Geometry check sheet. Reference: the model listing, model coordinates, mm. A direction names the side the tool comes from. Coordinates: 2 decimals unless noted, no trailing zeros. Write each loop counter-clockwise with the first axis right and the second up, starting at its lowest first coordinate (ties: lowest second). Pieces come first, ordered by that corner, then holes. Notation, with made-up numbers: (-12, 49.5) -> (47, 49.5) arc R12 cw to (47, 68.5) -> close; hole circle Ø10 at (44, 38.5). An arc over 180 degrees is marked (long way). Answer in a Markdown table with one row per item. Add a question column.
Q1. Section check B-B, the plane y = 15. Record the boundary of the cut face in (x, z), and give its area (3 significant figures).
Q2. Section check A-A, the plane z = -6.25. Record the boundary of the cut face in (x, y), and give its area (3 significant figures).
Q3. Tool access check on faces 1 (the face through (-27.488, -47.465, 0.246)), 2 (the face through (-21.883, 55.465, -9.616)), 3 (the face through (-29, 58, -8)), 4 (the face through (-25, 54, -21)), 5 (the face through (-24, -45, 0)). Record the directions out of +Z, -Z, +X, -X, +Y, -Y that give a thin tool (end or side, any length) a straight path to the whole face; none if there is none.
Q4. Thickness scan on line 1 (X direction, y = 54.45, z = 0); line 2 (Y direction, x = -26.5, z = -14); line 3 (Y direction, x = -21, z = -3.5). Record the ranges inside material, lowest first.
Q5. Release check for a two-part mould opening along Z. For faces 6 (the face through (-25, -50, 0)), 7 (the face through (-28.905, 3.165, 0.867)), 8 (the face through (-25, 55, -19)) record: pulls with the +Z half, pulls with the -Z half, needs draft (parallel to the pull), parting line crosses it, or undercut.
Q6. Gauge pin test, flat ends, axial feed: P1, Ø1.5, axis at y = -16.5, z = 0.5, coming from the +X side; P2, Ø12, axis at y = 7.5, z = -7, coming from the -X side; P3, Ø1.1, axis at x = -22, y = 6, coming from the -Z side; P4, Ø3, axis at x = -23.5, z = -14.5, coming from the +Y side. Record the tip position at first contact, or that the pin passes through.
```python
from build123d import *
from build123d.topology import SkipClean

# Parameters (mm, degrees)
SKETCH2_W                = 50
SKETCH2_H                = 90
BOSS_EXTRUDE1_DEPTH      = 1.5
BOSS_EXTRUDE2_DEPTH      = 45
BOSS_EXTRUDE2_DEPTH_BACK = 50
SKETCH3_R                = 4
BOSS_EXTRUDE3_DEPTH      = 3
BOSS_EXTRUDE4_DEPTH      = 5
SKETCH6_W                = 3
SKETCH6_H                = 90
CUT_EXTRUDE1_DEPTH       = 50
SKETCH7_R                = 2.5
BOSS_EXTRUDE5_DEPTH      = 5


with BuildPart() as part:
    # Sketch2 → Boss-Extrude1 (new, symmetric)
    with BuildSketch(Plane.XY):
        Rectangle(SKETCH2_W, SKETCH2_H)
    extrude(amount=BOSS_EXTRUDE1_DEPTH, both=True)

    # Sketch3 → Boss-Extrude2 (add, two sides: drawn at the far end of the back side and taken through both)
    with BuildSketch(Plane.XZ.offset(-BOSS_EXTRUDE2_DEPTH_BACK)):
        with Locations(Location((-25, 0, 0), (0, 0, 270))):
            Circle(SKETCH3_R)
    extrude(amount=BOSS_EXTRUDE2_DEPTH + BOSS_EXTRUDE2_DEPTH_BACK)

    # Sketch4 → Boss-Extrude3 (add)
    with BuildSketch(Plane(origin=(0, 50, 0), x_dir=(1, 0, 0), z_dir=(0, 1, 0))):
        with BuildLine():
            ThreePointArc((-30.45259438, 0.72056542), (-25, -5.5), (-19.54740562, 0.72056542))
            Line((-19.54740562, 0.72056542), (-20.881578947, 21))
            Line((-20.881578947, 21), (-29.118421053, 21))
            Line((-29.118421053, 21), (-30.45259438, 0.72056542))
        make_face()
    extrude(amount=BOSS_EXTRUDE3_DEPTH)

    # Sketch5 → Boss-Extrude4 (add)
    with SkipClean():  # the faces are left unmerged after this step: merging them gives an invalid solid
        with BuildSketch(Plane(origin=(0, 53, -53), x_dir=(1, 0, 0), z_dir=(0, -1, 0))):
            with BuildLine():
                Line((-30.5, 53), (-29.118421053, 32))
                Line((-29.118421053, 32), (-20.881578947, 32))
                Line((-20.881578947, 32), (-19.5, 53))
                ThreePointArc((-19.5, 53), (-25, 58.5), (-30.5, 53))
            make_face()
            with BuildLine():
                ThreePointArc((-28.717677987, 52.508705396), (-25, 56.75), (-21.282322013, 52.508705396))
                Line((-21.282322013, 52.508705396), (-22.5, 34))
                Line((-22.5, 34), (-27.5, 34))
                Line((-27.5, 34), (-28.717677987, 52.508705396))
            make_face(mode=Mode.SUBTRACT)
        extrude(amount=-BOSS_EXTRUDE4_DEPTH)

    # Sketch6 → Cut-Extrude1 (cut)
    with SkipClean():  # the faces are left unmerged after this step: merging them gives an invalid solid
        with BuildSketch(Plane(origin=(25, 0, 0), x_dir=(0, 0, -1), z_dir=(1, 0, 0))):
            Rectangle(SKETCH6_W, SKETCH6_H)
        extrude(amount=-CUT_EXTRUDE1_DEPTH, mode=Mode.SUBTRACT)

    # Sketch7 → Boss-Extrude5 (add)
    with SkipClean():  # the faces are left unmerged after this step: merging them gives an invalid solid
        with BuildSketch(Plane.XZ.offset(45)):
            with Locations(Location((-25, 0, 0), (0, 0, 36.869897646))):
                Circle(SKETCH7_R)
        extrude(amount=BOSS_EXTRUDE5_DEPTH)


solid = part.part
```
Calculated:
| question | item | result |
|---|---|---|
| 1 | outline | (-25, -1.5) -> (-25, 1.5) -> (-21.29, 1.5) arc R4 ccw (long way) to (-21.29, -1.5) -> close |
| 1 | area | 38.6 mm² |
| 2 | outline | (-30.09, 50) -> (-19.91, 50) -> (-19.91, 58) -> (-21.66, 58) -> (-21.66, 53) -> (-28.34, 53) -> (-28.34, 58) -> (-30.09, 58) -> close |
| 2 | area | 48.0 mm² |
| 3 | face 1 | -Y |
| 3 | face 2 | +Y |
| 3 | face 3 | +Z, -Z, +X, -X, +Y |
| 3 | face 4 | -Z, +X, -X, +Y, -Y |
| 3 | face 5 | +X |
| 4 | line 1 | x = -30.5 to -28.75, -21.25 to -19.5 |
| 4 | line 2 | y = 50 to 53 |
| 4 | line 3 | y = 50 to 58 |
| 5 | face 6 | needs draft |
| 5 | face 7 | parting line crosses it |
| 5 | face 8 | undercut |
| 6 | P1 | stops at x = -25 |
| 6 | P2 | stops at x = -28.87 |
| 6 | P3 | stops at z = -3.16 |
| 6 | P4 | stops at y = 58 |
